```python
from build123d import *

# Parameters (mm, degrees)
BOSS_EXTRUDE1_DEPTH = 24
SKETCH2_W           = 52
SKETCH2_H           = 93
CUT_EXTRUDE1_DEPTH  = 48
CUT_EXTRUDE2_DEPTH  = 105
SKETCH4_R           = 15
CUT_EXTRUDE3_DEPTH  = 105
SKETCH5_R           = 12
CUT_EXTRUDE4_DEPTH  = 105
FILLET1_R           = 1


with BuildPart() as part:
    # Sketch1 → Boss-Extrude1 (new, symmetric)
    with BuildSketch(Plane.XY):
        Polygon((-38, -49.5), (-26.452994616, -69.5), (26.452994616, -69.5), (38, -49.5), (38, 49.5), (-38, 49.5), align=None)
    extrude(amount=BOSS_EXTRUDE1_DEPTH, both=True)

    # Sketch2 → Cut-Extrude1 (cut)
    with BuildSketch(Plane.XY.offset(24)):
        with Locations((0, 3)):
            Rectangle(SKETCH2_W, SKETCH2_H)
    extrude(amount=-CUT_EXTRUDE1_DEPTH, mode=Mode.SUBTRACT)

    # Sketch3 → Cut-Extrude2 (cut)
    with BuildSketch(Plane.ZY.offset(38)):
        with BuildLine():
            Line((-24, 23.5), (-24, 49.5))
            Line((-24, 49.5), (24, 49.5))
            Line((24, 49.5), (24, 23.5))
            ThreePointArc((24, 23.5), (0, 47.5), (-24, 23.5))
        make_face()
    extrude(amount=-CUT_EXTRUDE2_DEPTH, mode=Mode.SUBTRACT)

    # Sketch4 → Cut-Extrude3 (cut)
    with BuildSketch(Plane.ZY.offset(38)):
        with Locations((0, 23.5)):
            Circle(SKETCH4_R)
    extrude(amount=-CUT_EXTRUDE3_DEPTH, mode=Mode.SUBTRACT)

    # Sketch5 → Cut-Extrude4 (cut)
    with BuildSketch(Plane(origin=(0, -43.5, 0), x_dir=(1, 0, 0), z_dir=(0, 1, 0))):
        with Locations(Location((0, 0, 0), (0, 0, 270))):
            Circle(SKETCH5_R)
    extrude(amount=-CUT_EXTRUDE4_DEPTH, mode=Mode.SUBTRACT)

    # Fillet1
    fillet1_edges = [part.edges().sort_by_distance(p)[0] for p in [
        (38, -49.5, 0),
        (26.452994616, -69.5, 0),
        (-26.452994616, -69.5, 0),
        (-38, -49.5, 0),
        (-32.226497308, -59.5, 24),
        (0, -69.5, 24),
        (32.226497308, -59.5, 24),
        (26, -10, -24),
        (0, -43.5, -24),
        (0, -43.5, 24),
        (26, -10, 24),
        (-26, -10, 24),
        (-26, -10, -24),
        (-26, 47.5, 0),
        (-38, -13, -24),
        (-38, -13, 24),
        (38, 47.5, 0),
        (26, 47.5, 0),
        (38, -13, 24),
        (-38, 47.5, 0),
        (32.226497308, -59.5, -24),
        (0, -69.5, -24),
        (-32.226497308, -59.5, -24),
        (0, -69.5, -12),
        (38, -13, -24),
    ]]
    fillet(fillet1_edges, radius=FILLET1_R)


solid = part.part
```
Can you work these out from the model? Positions are in its coordinate system, mm. A direction names the side the tool comes from. Round coordinates to 2 decimals unless told otherwise and drop trailing zeros. Order: outer loops, then holes, each group sorted by start corner. A loop starts at its lowest first (then second) coordinate and runs counter-clockwise, first axis right, second up.
(1) If we section it at C-C (z = 0): Count the separate pieces of the cut face and the enclosed holes in it, plus the area to 3 significant figures.
Results are:
separate pieces: 4
enclosed holes: 0
area: 2,580 mm2
(2) On a 3-axis mill with a long thin cutter (end or side, diameter ignored), from which of +Z, -Z, +X, -X, +Y, -Y can I reach the whole of each face in a straight line? I mean faces 1 (the face through (31.916, 8.857, -3.252)), 2 (the face through (-6, -43.5, 11)). Say none if no direction works.
Results are:
face 1: +X, -X
face 2: +Z, -Z, +Y
(3) If we section it at A-A (y = -13): Please give me the cut outline in (x, z), plus the area to 3 significant figures.
Results are:
outline: (-38, -23) arc R1 ccw to (-37, -24) - (-27, -24) arc R1 ccw to (-26, -23) - (-26, 23) arc R1 ccw to (-27, 24) - (-37, 24) arc R1 ccw to (-38, 23) - close; (26, -23) arc R1 ccw to (27, -24) - (37, -24) arc R1 ccw to (38, -23) - (38, 23) arc R1 ccw to (37, 24) - (27, 24) arc R1 ccw to (26, 23) - close
area: 1,150 mm2
(4) We'd pull the mould along Y, two halves only. Please class faces 3 (the face through (32.121, -59.081, 23.715)), 4 (the face through (-32.084, 8.857, -3.252)), 5 (the face through (31.93, 47.494, 0.528)): +Y half, -Y half, draft (parallel to the pull), parting line (faces both ways), or undercut.
Results are:
face 3: -Y half
face 4: undercut
face 5: +Y half
(5) I'm going to push flat-ended pins straight in: pin 1 (3 mm diameter, centred on x = 26.5, z = -16, fed in from +Y); pin 2 (1 mm diameter, centred on x = -28.5, z = 12, fed in from +Y); pin 3 (14.5 mm diameter, centred on x = 0, z = 0, fed in from +Y) (1 decimal); pin 4 (2 mm diameter, centred on y = -56, z = -17, fed in from -X). Where does each tip first touch, or does it pass through?
Results are:
pin 1: stops at y = 42.58
pin 2: stops at y = 44.57
pin 3: passes through
pin 4: stops at x = -34.82
(6) If I drill on L1, parallel to X at y = -42, z = -11; L2, parallel to X at y = -48.75, z = 0; L3, parallel to Y at x = -30.25, z = 0, over which ranges is the centre line in solid material (lowest first)?
Results are:
L1: x = -38 to -26, 26 to 38
L2: x = -38 to -12, 12 to 38
L3: y = -62.92 to 8.5, 38.5 to 47.5
(7) If we section it at B-B (x = 0): Please give me the cut outline in (y, z), plus the area to 3 significant figures.
Results are:
outline: (-69.5, -23) arc R1 ccw to (-68.5, -24) - (-44.5, -24) arc R1 ccw to (-43.5, -23) - (-43.5, -12) - (-68.5, -12) arc R1 ccw to (-69.5, -13) - close; (-69.5, 13) arc R1 ccw to (-68.5, 12) - (-43.5, 12) - (-43.5, 23) arc R1 ccw to (-44.5, 24) - (-68.5, 24) arc R1 ccw to (-69.5, 23) - close
area: 623 mm2
